```python
from build123d import *

# Parameters (mm, degrees)
EXTRUDE_THIN1_DEPTH = 52
SKETCH2_R           = 10
CUT_EXTRUDE2_DEPTH  = 10
FILLET1_R           = 30
CUT_EXTRUDE3_DEPTH  = 10
FILLET2_R           = 10
SKETCH4_R           = 5
CUT_EXTRUDE4_DEPTH  = 10


with BuildPart() as part:
    # Sketch1 → Extrude-Thin1 (new body)
    with BuildSketch(Plane.XY):
        Polygon((17.101007166, 46.984631039), (0, 0), (60, 0), (117.955549577, -15.529142706), (120.543740028, -5.869884443), (61.316524976, 10), (14.281480067, 10), (26.497933374, 43.564429606), align=None)
    extrude(amount=EXTRUDE_THIN1_DEPTH)

    # Sketch2 → Cut-Extrude2 (cut)
    with BuildSketch(Plane(origin=(0, 0, 0), x_dir=(0, 0, 1), z_dir=(-0.9396926207859096, 0.34202014332566566, 0))):
        with Locations(Location((25.484668599, 30, 0), (0, 0, 270))):
            Circle(SKETCH2_R)
    extrude(amount=-CUT_EXTRUDE2_DEPTH, mode=Mode.SUBTRACT)

    # Fillet1
    # the kernel refuses this fillet: 30 mm, written as the material it takes off along each edge
    with BuildSketch(Plane(origin=(96.974879933, 17.912918857, 0), x_dir=(0, 0, 1), z_dir=(-0.9396926207859095, 0.34202014332566577, 0))) as fillet1_piece_1_section:
        with BuildLine():
            CenterArc((FILLET1_R, -FILLET1_R), FILLET1_R, 90, 90)
            Line((0, -FILLET1_R), (0, 0))
            Line((0, 0), (FILLET1_R, 0))
        make_face()
    fillet1_piece_1 = extrude(amount=160, mode=Mode.PRIVATE)
    fillet1_piece_1 = split(fillet1_piece_1, bisect_by=Plane(origin=(19.547189191, 10, 6.743574493), z_dir=(0, 1, 0)), keep=Keep.TOP, mode=Mode.PRIVATE)
    add(fillet1_piece_1, mode=Mode.SUBTRACT)
    with BuildSketch(Plane(origin=(96.974879933, 17.912918857, 52), x_dir=(0, 0, -1), z_dir=(-0.9396926207859095, 0.34202014332566577, 0))) as fillet1_piece_2_section:
        with BuildLine():
            CenterArc((FILLET1_R, FILLET1_R), FILLET1_R, 180, 90)
            Line((0, FILLET1_R), (0, 0))
            Line((0, 0), (FILLET1_R, 0))
        make_face()
    fillet1_piece_2 = extrude(amount=160, mode=Mode.PRIVATE)
    fillet1_piece_2 = split(fillet1_piece_2, bisect_by=Plane(origin=(19.547189191, 10, 45.256425507), z_dir=(0, 1, 0)), keep=Keep.TOP, mode=Mode.PRIVATE)
    add(fillet1_piece_2, mode=Mode.SUBTRACT)

    # Sketch3 → Cut-Extrude3 (cut)
    with BuildSketch(Plane(origin=(6.607428337, 24.659258263, 0), x_dir=(0.9659258262890682, -0.25881904510252124, 0), z_dir=(0.25881904510252124, 0.9659258262890682, 0))):
        with BuildLine():
            Line((90.180356015, -36), (90.180356015, -16))
            ThreePointArc((90.180356015, -16), (96.639024601, -9.541331414), (103.097693188, -16))
            Line((103.097693188, -16), (103.097693188, -36))
            ThreePointArc((103.097693188, -36), (96.639024601, -42.458668586), (90.180356015, -36))
        make_face()
    extrude(amount=-CUT_EXTRUDE3_DEPTH, mode=Mode.SUBTRACT)

    # Fillet2
    fillet2_edges = [part.edges().sort_by_distance(p)[0] for p in [
        (119.249644803, -10.699513575, 52),
        (119.249644803, -10.699513575, 0),
    ]]
    fillet(fillet2_edges, radius=FILLET2_R)

    # Sketch4 → Cut-Extrude4 (cut)
    with BuildSketch(Plane(origin=(0, 10, 0), x_dir=(1, 0, 0), z_dir=(0, 1, 0))):
        with Locations(Location((29.281480067, -43.506992199, 0), (0, 0, 270))):
            Circle(SKETCH4_R)
        with Locations(Location((29.281480067, -13.135621251, 0), (0, 0, 270))):
            Circle(SKETCH4_R)
        with Locations(Location((46.316524976, -13.135621251, 0), (0, 0, 270))):
            Circle(SKETCH4_R)
        with Locations(Location((46.316524976, -43.506992199, 0), (0, 0, 270))):
            Circle(SKETCH4_R)
    extrude(amount=-CUT_EXTRUDE4_DEPTH, mode=Mode.SUBTRACT)


solid = part.part
```
The model under review builds one solid part; all positions refer to its coordinate system, in mm. A direction names the side the tool comes from. Coordinates: 2 decimals unless noted, no trailing zeros. Order: outer loops, then holes, each group sorted by start corner. A loop starts at its lowest first (then second) coordinate and runs counter-clockwise, first axis right, second up. Notation, with made-up numbers: (-18, -20) -> (-4, -20) arc R21 cw to (-4, 4) -> close; hole circle Ø5 at (-36, -29). An arc over 180 degrees is marked (long way). Answer in a Markdown table with one row per item. Add a question column.
Item 1: We need section D-D on x = 54. Write out the cut boundary in (y, z).
Item 2: We need section B-B on z = 44. Write out the cut boundary in (x, y).
Item 3: To check wall thickness, follow probe 1 along Y at (x, z) = (20.5, 31); probe 2 along Y at (x, z) = (33, 4); probe 3 along Z at (x, y) = (50.5, 5.5). State the ranges of each line that lie inside material, in increasing order.
Item 4: We need section C-C on y = 2.5. Write out the cut boundary in (x, z), plus the area to 3 significant figures.
Item 5: We need section A-A on x = 28. Write out the cut boundary in (y, z).
Item 6: Mouldability with a two-part tool opening along Y and no side actions: class faces 4 (the flat face through (88.572, -7.656, 25.636)), 5 (the flat face through (55, 2, 52)), 6 (the flat face through (16.217, 15.319, 19.858)) as +Y half, -Y half, draft (parallel to the pull), parting line (faces both ways), or undercut.
Item 7: Clearance check with flat-ended pins moving along their axes: pin 1 (4 mm diameter, centred on y = -6.5, z = 7, fed in from +X); pin 2 (6 mm diameter, centred on x = 94.5, z = 33.5, fed in from +Y); pin 3 (16 mm diameter, centred on x = 29.28, z = 13.14, fed in from -Y). State where each tip first meets the part, or that it passes through.
Item 8: Machinability: for faces 1 (the cylindrical face through (98.54, -5.078, 9.543)), 2 (the cylindrical face through (33.5, 5.07, 15.82)), 3 (the flat face through (38, 10, 26)), which of the approach directions +Z, -Z, +X, -X, +Y, -Y give a long, thin tool a straight path to every point of the face, cutting with its end or side? Answer none if there is none.
Final values:
| question | item | result |
|---|---|---|
| 1 | outline | (0, 0) -> (10, 0) -> (10, 52) -> (0, 52) -> close |
| 2 | outline | (0, 0) -> (24.31, 0) -> (24.31, 10) -> (14.28, 10) -> (23.21, 34.54) -> (13.82, 37.96) -> close; (34.26, 0) -> (41.34, 0) -> (41.34, 10) -> (34.26, 10) -> close; (51.29, 0) -> (60, 0) -> (117.76, -15.48) -> (120.35, -5.82) -> (61.32, 10) -> (51.29, 10) -> close |
| 3 | probe 1 | y = 0 to 10, 33.34 to 44.28 |
| 3 | probe 2 | y = 0 to 10 |
| 3 | probe 3 | z = 0 to 10.4, 15.87 to 40.77, 46.25 to 52 |
| 4 | outline | (0.91, 0) -> (89.31, 0) -> (89.31, 52) -> (0.91, 52) -> close; hole circle Ø10 at (29.28, 13.14); hole circle Ø10 at (29.28, 43.51); hole circle Ø10 at (46.32, 13.14); hole circle Ø10 at (46.32, 43.51) |
| 4 | area | 4,280 mm2 |
| 5 | outline | (0, 0) -> (10, 0) -> (10, 8.3) -> (0, 8.3) -> close; (0, 17.97) -> (10, 17.97) -> (10, 38.67) -> (0, 38.67) -> close; (0, 48.34) -> (10, 48.34) -> (10, 52) -> (0, 52) -> close |
| 6 | face 4 | -Y half |
| 6 | face 5 | draft |
| 6 | face 6 | undercut |
| 7 | pin 1 | stops at x = 120.48 |
| 7 | pin 2 | stops at y = 1.91 |
| 7 | pin 3 | stops at y = 0 |
| 8 | face 1 | none |
| 8 | face 2 | -Y |
| 8 | face 3 | +Z, -Z, +X |
